The model under review builds one solid part; all positions refer to its coordinate system, in mm. Give positions to 0.01 mm unless a question says otherwise; leave off trailing zeros. Order: outer loops, then holes, each group sorted by start corner. A loop starts at its lowest first (then second) coordinate and runs counter-clockwise, first axis right, second up. Notation, with made-up numbers: (17, -9.5) -> (49, -9.5) arc R8 cw to (49, -0.5) -> close; hole circle Ø9 at (-24.5, -16). An arc over 180 degrees is marked (long way). Use one line per item in the form item = value.
Autodesk Inventor part; units mm, degrees
ref_plane "YZ Plane" through (0, 0, 0) normal (1, 0, 0) x (0, 1, 0)
ref_plane "XZ Plane" through (0, 0, 0) normal (0, 1, 0) x (-1, 0, 0)
ref_plane "XY Plane" through (0, 0, 0) normal (0, 0, 1) x (1, 0, 0)
sketch "Sketch1" plane through (0, 0, 0) normal (0, 0, 1) x (1, 0, 0)
  circle A0 centre (0, 0) radius 76.2
  dimension "d0" = 152.4
extrude "Extrusion1" add sketch "Sketch1" along normal mid plane 6.35
sketch "Sketch3" plane through (0, 0, 3.175) normal (0, 0, 1) x (1, 0, 0)
  circle A0 centre (0, 0) radius 25.4
  dimension "d8" = 50.8
extrude "Extrusion3" cut sketch "Sketch3" against normal through all
sketch "Sketch5" plane through (0, 0, 3.175) normal (0, 0, 1) x (1, 0, 0)
  arc A0 (3.175, 25.2008) -> (-3.175, 25.2008) centre (0, 0) ccw
  circle A1 centre (0, 0) radius 25.4
  line L0 (-3.175, 25.2008) -> (-3.175, 22.225)
  line L1 (3.175, 25.2008) -> (3.175, 22.225)
  line L2 (-3.175, 22.225) -> (3.175, 22.225)
  dimension "d11" = 3.175
  dimension "d13" = 6.35
extrude "Extrusion4" add sketch "Sketch5" against normal blind 6.35 contours L1 L2 L0 A0
sketch "Sketch7" plane through (0, 0, -3.175) normal (0, 0, -1) x (-1, 0, 0)
  arc A0 (3.175, -25.2008) -> (20.237, -15.35) centre (0, 0) ccw
  circle A1 centre (0, 0) radius 38.1
  circle A2 centre (0, 0) radius 4.7625
  dimension "d19" = 76.2
  dimension "d20" = 9.525
properties part number "6x1_4-testSampleGear" material "PC/ABS Plastic"
1. Add section C-C on z = -1.75. Give the boundary of the cut face in (x, y) (3 decimals), then the cut area to 3 significant figures.
Values:
outline = circle Ø152.4 at (0, 0); hole (-3.175, 22.225) -> (-3.175, 25.201) arc R25.4 ccw (long way) to (3.175, 25.201) -> (3.175, 22.225) -> close
area = 16,200 mm^2
2. Add section D-D on y = 32. Give the boundary of the cut face in (x, z) (3 decimals).
Values:
outline = (-69.155, -3.175) -> (69.155, -3.175) -> (69.155, 3.175) -> (-69.155, 3.175) -> close
3. For pin 1 Ø0.9 at (y, z) = (24, -1) entering from +X; pin 2 Ø3.5 at (y, z) = (24, 0) entering from -X; pin 3 Ø3 at (y, z) = (-14, 2) entering from -X, all flat-tipped, find the tip position at first contact; note any pin that passes through.
Values:
pin_1 = 72.47
pin_2 = -72.88
pin_3 = -75.17
4. The part is to be moulded in two halves that separate along X. For faces 1 (the face through (-60.47, 46.367, -0.044)), 2 (the face through (33, 1, 3.175)), 3 (the face through (0, 22.225, 0)), say which applies: +X half, -X half, draft (parallel to the pull), parting line (faces both ways), or undercut.
Values:
face_1 = parting line
face_2 = draft
face_3 = undercut
5. For L1, parallel to Y at x = 0, z = 1 (3 decimals); L2, parallel to Y at x = 21, z = -0.5; L3, parallel to X at y = -19, z = 2.5, list the stretches that pass through material, from the lowest coordinate up.
Values:
L1 = -76.2 to -25.4, 22.225 to 76.2
L2 = -73.25 to -14.29, 14.29 to 73.25
L3 = -73.79 to -16.86, 16.86 to 73.79
6. Add section A-A on x = 0. Give the boundary of the cut face in (y, z) (3 decimals), then the cut area to 3 significant figures.
Values:
outline = (-76.2, -3.175) -> (-25.4, -3.175) -> (-25.4, 3.175) -> (-76.2, 3.175) -> close; (22.225, -3.175) -> (76.2, -3.175) -> (76.2, 3.175) -> (22.225, 3.175) -> close
area = 665 mm^2
7. Add section B-B on y = 0. Give the boundary of the cut face in (x, z) (3 decimals), then the cut area to 3 significant figures.
Values:
outline = (-76.2, -3.175) -> (-25.4, -3.175) -> (-25.4, 3.175) -> (-76.2, 3.175) -> close; (25.4, -3.175) -> (76.2, -3.175) -> (76.2, 3.175) -> (25.4, 3.175) -> close
area = 645 mm^2
